from build123d import *

# Parameters (mm, degrees)
SKETCH1_R           = 14
SKETCH1_R_2         = 6
SKETCH1_R_3         = 1.5
BOSS_EXTRUDE1_DEPTH = 5
CHAMFER1_SIZE       = 0.25


with BuildPart() as part:
    # Sketch1 → Boss-Extrude1 (new body, symmetric)
    with BuildSketch(Plane.XY):
        Circle(SKETCH1_R)
        Circle(SKETCH1_R_2, mode=Mode.SUBTRACT)
        with Locations((0, 10)):
            Circle(SKETCH1_R_3, mode=Mode.SUBTRACT)
        with Locations((8.660254038, -5)):
            Circle(SKETCH1_R_3, mode=Mode.SUBTRACT)
        with Locations((-8.660254038, -5)):
            Circle(SKETCH1_R_3, mode=Mode.SUBTRACT)
    extrude(amount=BOSS_EXTRUDE1_DEPTH, both=True)

    # Chamfer1
    chamfer1_edges = [part.edges().sort_by_distance(p)[0] for p in [
        (-14, 0, -5),
        (-14, 0, 5),
        (-6, 0, -5),
        (-6, 0, 5),
    ]]
    chamfer(chamfer1_edges, length=CHAMFER1_SIZE)


solid = part.part
Source: CAD feature listing. Evaluate the final solid. Frame: model axes, mm. Round coordinates to 2 decimals unless told otherwise and drop trailing zeros. Order: outer loops, then holes, each group sorted by start corner. A loop starts at its lowest first (then second) coordinate and runs counter-clockwise, first axis right, second up. Notation, with made-up numbers: (44.5, -20.75) - (94.5, -20.75) arc R20 ccw to (94.5, -16.75) - close; hole circle Ø1 at (48, 53.5). An arc over 180 degrees is marked (long way). Use a Markdown table: item, result. Add a question column.
1. First-contact query: pin 1 (5 mm diameter, centred on y = -3, z = 1.5, fed in from +X); pin 2 (5 mm diameter, centred on y = -5.5, z = -3, fed in from +X). Flat tips, straight axial feed; report the tip coordinate or a pass-through.
2. Section query B-B (x = 0). Return the cut outline in (y, z).
3. Section query A-A (y = 0). Return the cut outline in (x, z).
4. Section query C-C (z = 3.75). Return the cut outline in (x, y).
5. Section query D-D (y = -5). Give the number of separate pieces and of enclosed holes in the cut face, then the cut area to 3 significant figures.
6. Line query: probe 1 along Y at (x, z) = (0, 0.5); probe 2 along Y at (x, z) = (1.25, -2.75); probe 3 along X at (y, z) = (-0.5, 1). Output: solid intervals per line, ascending.
7. Mould query, pull axis Y, two halves, no side actions, for faces 1 (the flat face through (6, -3, 5)), 2 (the cylindrical face through (-6, 0, 0)), 3 (the cylindrical face through (12.932, -5.362, 0.067)). Classes: +Y half, -Y half, draft (parallel to the pull), parting line (faces both ways), or undercut.
Derived:
| question | item | result |
|---|---|---|
| 1 | pin 1 | x = 13.99 |
| 1 | pin 2 | x = 13.67 |
| 2 | outline | (-14, -4.75) - (-13.75, -5) - (-6.25, -5) - (-6, -4.75) - (-6, 4.75) - (-6.25, 5) - (-13.75, 5) - (-14, 4.75) - close; (6, -4.75) - (6.25, -5) - (8.5, -5) - (8.5, 5) - (6.25, 5) - (6, 4.75) - close; (11.5, -5) - (13.75, -5) - (14, -4.75) - (14, 4.75) - (13.75, 5) - (11.5, 5) - close |
| 3 | outline | (-14, -4.75) - (-13.75, -5) - (-6.25, -5) - (-6, -4.75) - (-6, 4.75) - (-6.25, 5) - (-13.75, 5) - (-14, 4.75) - close; (6, -4.75) - (6.25, -5) - (13.75, -5) - (14, -4.75) - (14, 4.75) - (13.75, 5) - (6.25, 5) - (6, 4.75) - close |
| 4 | outline | circle Ø28 at (0, 0); hole circle Ø3 at (-8.66, -5); hole circle Ø12 at (0, 0); hole circle Ø3 at (0, 10); hole circle Ø3 at (8.66, -5) |
| 5 | separate pieces | 4 |
| 5 | enclosed holes | 0 |
| 5 | area | 135 mm2 |
| 6 | probe 1 | -14 to -6, 6 to 8.5, 11.5 to 14 |
| 6 | probe 2 | -13.94 to -5.87, 5.87 to 9.17, 10.83 to 13.94 |
| 6 | probe 3 | -13.99 to -5.98, 5.98 to 13.99 |
| 7 | face 1 | draft |
| 7 | face 2 | undercut |
| 7 | face 3 | parting line |
